from build123d import *

# Parameters (mm, degrees)
F1_DEPTH = 7
F3_DEPTH = 1
F5_DEPTH = 1


with BuildPart() as f1:
    # F0 (on Front) → F1 (new body)
    with BuildSketch(Plane.XZ):
        Polygon((0, 8), (0, 0), (10, 0), (10, 8), (9, 8), (9, 6), (9.1, 6), (9.1, 5.6), (0.9, 5.6), (0.9, 6), (1, 6), (1, 8), align=None)
    extrude(amount=F1_DEPTH)

    # F2 (on face) → F3 (join)
    with BuildSketch(Plane.XZ.offset(7)):
        Polygon((1, 8), (0, 8), (0, 0), (10, 0), (10, 8), (9, 8), (9, 6), (9.1, 6), (9.1, 5.6), (0.9, 5.6), (0.9, 6), (1, 6), align=None)
        Polygon((9, 8), (1, 8), (1, 6), (0.9, 6), (0.9, 5.6), (9.1, 5.6), (9.1, 6), (9, 6), align=None)
    extrude(amount=F3_DEPTH)

    # F4 (on face) → F5 (join)
    with BuildSketch(Plane(origin=(0, 0, 0), x_dir=(-1, 0, 0), z_dir=(0, 1, 0))):
        Polygon((-9, 8), (-10, 8), (-10, 0), (0, 0), (0, 8), (-1, 8), (-1, 6), (-0.9, 6), (-0.9, 5.6), (-9.1, 5.6), (-9.1, 6), (-9, 6), align=None)
        Polygon((-1, 8), (-9, 8), (-9, 6), (-9.1, 6), (-9.1, 5.6), (-0.9, 5.6), (-0.9, 6), (-1, 6), align=None)
    extrude(amount=F5_DEPTH)


solid = f1.part
Source: CAD feature listing. Evaluate the final solid. Frame: model axes, mm. A direction names the side the tool comes from. Give positions to 0.01 mm unless a question says otherwise; leave off trailing zeros. Write each loop counter-clockwise with the first axis right and the second up, starting at its lowest first coordinate (ties: lowest second). Pieces come first, ordered by that corner, then holes. Notation, with made-up numbers: M 37,-7.75 L 54,-7.75 A5 cw 54,-0.75 Z; hole C 53.5,48.5 d6. An arc over 180 degrees is marked long. Return JSON: item names as keys, results as strings. Group by question number.
1) Cut plane A-A, the plane x = 8.75. Output: boundary loops of the cut face in (y, z).
2) First-contact query: pin 1 Ø2 at (y, z) = (-6, 4.5) entering from -X; pin 2 Ø3.5 at (x, y) = (4.5, -4) entering from +Z. Flat tips, straight axial feed; report the tip coordinate or a pass-through.
3) Cut plane C-C, the plane z = 7.75. Output: boundary loops of the cut face in (x, y), then the cut area to 3 significant figures.
4) Cut plane B-B, the plane y = -4.75. Output: boundary loops of the cut face in (x, z).
5) Draft query along X for faces 1 (the face through (10, -4, 4)), 2 (the face through (5, -3, 5.6)), 3 (the face through (0, -4, 4)). Return one class per face: released by +X, released by -X, zero draft, split by the parting line, or undercut.
6) Set-up query: faces 4 (the face through (5, 1, 4)), 5 (the face through (1, -3, 7)). Return all of +Z, -Z, +X, -X, +Y, -Y with unobstructed straight access to the full face (end or side cutting, diameter ignored); none if empty.
7) Ray query, L1, parallel to Y at x = 2, z = 5.75; L2, parallel to X at y = -0.5, z = 7; L3, parallel to Z at x = 2, y = -2. Return the intervals inside material, ascending.
Data:
{
 "1": {"outline": "M -8,0 L 1,0 L 1,8 L 0,8 L 0,5.6 L -7,5.6 L -7,8 L -8,8 Z"},
 "2": {"pin 1": "stops at x = 0", "pin 2": "stops at z = 5.6"},
 "3": {"outline": "M 0,-8 L 10,-8 L 10,1 L 0,1 Z; hole M 1,-7 L 9,-7 L 9,0 L 1,0 Z", "area": "34.0 mm²"},
 "4": {"outline": "M 0,0 L 10,0 L 10,8 L 9,8 L 9,6 L 9.1,6 L 9.1,5.6 L 0.9,5.6 L 0.9,6 L 1,6 L 1,8 L 0,8 Z"},
 "5": {"face 1": "released by +X", "face 2": "undercut", "face 3": "released by -X"},
 "6": {"face 4": "+Z, -Z, +X, -X, +Y", "face 5": "+Z"},
 "7": {"L1": "y = -8 to -7, 0 to 1", "L2": "x = 0 to 1, 9 to 10", "L3": "z = 0 to 5.6"}
}
